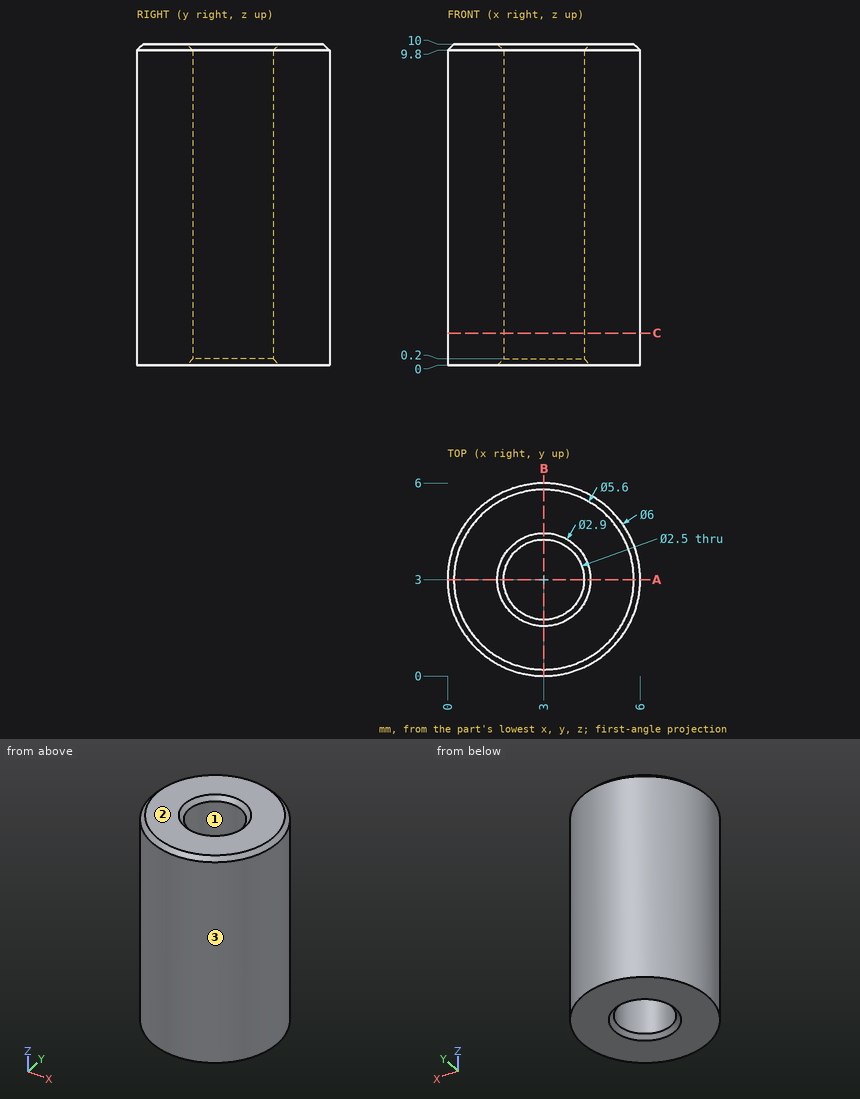
Job drawing, mm, ordinate dimensions from the low corner. One solid piece. Round coordinates to 2 decimals unless told otherwise and drop trailing zeros. Write each loop counter-clockwise with the first axis right and the second up, starting at its lowest first coordinate (ties: lowest second). Pieces come first, ordered by that corner, then holes.
1) Drill centre lines: probe 1 along Y at (x, z) = (3, 5); probe 2 along X at (y, z) = (3.65, 3.5); probe 3 along X at (y, z) = (3.95, 4.25). Where is each one in solid material? Low to high.
2) Band-saw the part on A-A, the plane y = 3. List the corners of the cut face in (x, z).
3) Mould opens along Y. For the marked faces 1, 2 and 3 say: +Y half, -Y half, draft (parallel to the pull), parting line (faces both ways), or undercut.
4) Band-saw the part on C-C, the plane z = 1. List the corners of the cut face in (x, y).
5) Pin check, flat tips, straight feed: pin 1 (1 mm diameter, centred on y = 1, z = 7, fed in from -X); pin 2 (3 mm diameter, centred on x = 1, z = 8, fed in from -Y); pin 3 (1 mm diameter, centred on x = 2, z = 8, fed in from +Y). Stop position of each tip, or through.
Ans:
1. probe 1: y = 0 to 1.75, 4.25 to 6
1. probe 2: x = 0.07 to 1.93, 4.07 to 5.93
1. probe 3: x = 0.15 to 2.19, 3.81 to 5.85
2. outline: (0, 0) - (1.55, 0) - (1.75, 0.2) - (1.75, 9.8) - (1.55, 10) - (0.2, 10) - (0, 9.8) - close; (4.25, 0.2) - (4.45, 0) - (6, 0) - (6, 9.8) - (5.8, 10) - (4.45, 10) - (4.25, 9.8) - close
3. face 1: undercut
3. face 2: draft
3. face 3: parting line
4. outline: circle Ø6 at (3, 3); hole circle Ø2.5 at (3, 3)
5. pin 1: stops at x = 0.4
5. pin 2: stops at y = 0.04
5. pin 3: stops at y = 5.96
